Autodesk Inventor part; units mm, degrees
ref_plane "YZ Plane" through (0, 0, 0) normal (1, 0, 0) x (0, 1, 0)
ref_plane "XZ Plane" through (0, 0, 0) normal (0, 1, 0) x (-1, 0, 0)
ref_plane "XY Plane" through (0, 0, 0) normal (0, 0, 1) x (1, 0, 0)
sketch "Эскиз1" plane through (0, 0, 0) normal (0, 0, 1) x (1, 0, 0)
  line L0 (0, 0) -> (28.3511, 0) construction
  line L1 (0, 20) -> (0, 0)
  line L2 (1, 21) -> (5, 21)
  arc A0 (1, 21) -> (0, 20) centre (1, 20) ccw
  line L3 (5, 26) -> (1, 26)
  arc A1 (1, 26) -> (-5, 20) centre (1, 20) ccw
  line L4 (-5, 20) -> (-5, 0)
  line L5 (-5, 0) -> (3.5853, 0) construction
  line L6 (5, 26) -> (5, 21)
  line L7 (-5, 0) -> (0, 0)
  dimension "d0" = 42
  dimension "d1" = 1
  dimension "d2" = 5
  dimension "d3" = 52
  dimension "d5" = 10
revolve "Вращение1" add sketch "Эскиз1" angle 360 about axis through (0, 0, 0) along (1, 0, 0)
properties part number "Регулировка"
Could you check a few things on this model? Use its own coordinates, in mm. Round coordinates to 2 decimals unless told otherwise and drop trailing zeros. Loops run counter-clockwise (first coordinate to the right, second up) from the corner with the lowest first, then second, coordinate; pieces in that order, holes last. Notation, with made-up numbers: (-21, -5.5) - (38, -5.5) arc R35 cw to (38, 29.5) - close; hole circle Ø9 at (-11.5, -28.75). An arc over 180 degrees is marked (long way). Answer in a Markdown table with one row per item. Add a question column.
(1) If we section it at C-C (x = 4.25): Please give me the cut outline in (y, z), plus the area to 3 significant figures.
(2) I need wall thicknesses on line 1 along Z through (x, y) = (2.1, 0); line 2 along X through (y, z) = (10, 17); line 3 along Y through (x, z) = (1.5, 17). Which ranges of each line are inside material? Lowest first, please.
(3) If we mould it in two halves opening along Y, with no side actions, what happens to faces 1 (the face through (0, 0, 0)), 2 (the face through (3.03, 20.03, 6.31)), 3 (the face through (2.972, -20.633, 15.821)), 4 (the face through (-5, 0, 0))? For each: pulls with the +Y half, pulls with the -Y half, needs draft (parallel to the pull), parting line crosses it, or undercut.
(4) If we section it at A-A (z = 0): Please give me the cut outline in (x, y), plus the area to 3 significant figures.
(5) I'm going to push flat-ended pins straight in: pin 1 (25 mm diameter, centred on y = 0, z = 0, fed in from +X); pin 2 (6 mm diameter, centred on x = -1, z = -18, fed in from +Y); pin 3 (2 mm diameter, centred on x = 0, z = -16.5, fed in from -Y). Where does each tip first touch, or does it pass through?
Model answer:
| question | item | result |
|---|---|---|
| 1 | outline | circle Ø52 at (0, 0); hole circle Ø42 at (0, 0) |
| 1 | area | 738 mm² |
| 2 | line 1 | z = -26 to -21, 21 to 26 |
| 2 | line 2 | x = -5 to 0 |
| 2 | line 3 | y = -19.67 to -12.33, 12.33 to 19.67 |
| 3 | face 1 | undercut |
| 3 | face 2 | undercut |
| 3 | face 3 | parting line crosses it |
| 3 | face 4 | needs draft |
| 4 | outline | (-5, -20) arc R6 ccw to (1, -26) - (5, -26) - (5, -21) - (1, -21) arc R1 cw to (0, -20) - (0, 20) arc R1 cw to (1, 21) - (5, 21) - (5, 26) - (1, 26) arc R6 ccw to (-5, 20) - close |
| 4 | area | 295 mm² |
| 5 | pin 1 | stops at x = 0 |
| 5 | pin 2 | stops at y = 21.01 |
| 5 | pin 3 | stops at y = -20.79 |
